```python
from build123d import *

# Parameters (mm, degrees)
F3_DEPTH = 34
F4_DEPTH = 18.001
F6_D     = 20
F7_R     = 7.5
F8_DEPTH = 5


with BuildPart() as f3:
    # F0 (on Front) → F3 (new body)
    with BuildSketch(Plane.XZ):
        Polygon((-55, 15), (-55, 0), (34, 0), (34, 18), (22, 18), (19, 15), align=None)
    extrude(amount=F3_DEPTH)

    # F1 (on Top) → F4 (intersect, through all)
    with BuildSketch(Plane.XY):
        Polygon((16, 0), (-55, 0), (-55, -10), (0, -34), (34, -34), (34, -24), (16, -24), align=None)
    extrude(amount=F4_DEPTH, mode=Mode.INTERSECT)

    # F5: F3 across plane


with BuildPart() as f3_1:
    add(f3.part)
    add(f3.part.mirror(Plane.XZ))

    # F6 (through all)
    with Locations(Plane(origin=(0, 0, 0), x_dir=(1, 0, 0), z_dir=(0, 0, -1))):
        with Locations((0, 0)):
            Hole(F6_D / 2)

    # F7 (on face) → F8 (cut)
    with BuildSketch(Plane.XY.offset(15)):
        with Locations((-45, 0)):
            Circle(F7_R)
    extrude(amount=-F8_DEPTH, mode=Mode.SUBTRACT)


solid = f3_1.part
```
The listing builds one solid part. Answer for the finished solid, in the listing's coordinates (mm). A direction names the side the tool comes from. Round coordinates to 2 decimals unless told otherwise and drop trailing zeros. Order: outer loops, then holes, each group sorted by start corner. A loop starts at its lowest first (then second) coordinate and runs counter-clockwise, first axis right, second up. Notation, with made-up numbers: (69, 12) -> (124, 12) arc R29 ccw to (124, 37) -> close; hole circle Ø6 at (30, 32.5). An arc over 180 degrees is marked (long way). Answer as CSV lines item,"result". Start each with the question number.
(1) The part is cut by section B-B (x = 23). Determine the outline of the cut face in (y, z), then the cut area to 3 significant figures.
(2) The part is cut by section A-A (y = 6). Determine the outline of the cut face in (x, z).
(3) A tool of negligible diameter and unlimited length cuts with its end or side. For faces 5 (the face through (34, -29, 9)), 6 (the face through (-17, 0, 15)), 7 (the face through (25, -24, 9)), from which of +Z, -Z, +X, -X, +Y, -Y can it reach the whole face along a straight path? Write none if from no direction.
(4) Flat-ended cylindrical pins translate along their axes: pin 1 Ø8 at (x, z) = (-36, 15) entering from +Y; pin 2 Ø12 at (x, y) = (0, 0) entering from +Z; pin 3 Ø20.5 at (x, y) = (-3, -13.5) entering from +Z; pin 4 Ø2 at (y, z) = (-26, 10.5) entering from -X (3 decimals). Find the tip coordinate at first contact, or state that the pin passes through.
(5) For a pull along X with two mould halves and no side action, classify faces 1 (the face through (-45, 0, 10)), 2 (the face through (28, 29, 18)), 3 (the face through (16, 0, 7)), 4 (the face through (-37.846, 2.253, 12.535)) as +X half, -X half, draft (parallel to the pull), parting line (faces both ways), or undercut.
(6) The part is cut by section D-D (z = 3). Determine the outline of the cut face in (x, y).
(7) The part is cut by section C-C (z = 13.75). Determine the outline of the cut face in (x, y).
(8) Find the intervals of material crossed by probe 1 along Y at (x, z) = (22.5, 13.5); probe 2 along Y at (x, z) = (0, 8); probe 3 along Z at (x, y) = (-9, 14), in increasing order. Write a range as from..to.
Evaluation:
1,outline,"(-34, 0) -> (-24, 0) -> (-24, 18) -> (-34, 18) -> close; (24, 0) -> (34, 0) -> (34, 18) -> (24, 18) -> close"
1,area,"360 mm²"
2,outline,"(-55, 0) -> (-8, 0) -> (-8, 15) -> (-40.5, 15) -> (-40.5, 10) -> (-49.5, 10) -> (-49.5, 15) -> (-55, 15) -> close; (8, 0) -> (16, 0) -> (16, 15) -> (8, 15) -> close"
3,face 5,"+Z, -Z, +X, +Y, -Y"
3,face 6,"+Z, -X, +Y, -Y"
3,face 7,"+Z, -Z, +X"
4,pin 1,"y = 20.04"
4,pin 2,"through"
4,pin 3,"z = 15"
4,pin 4,"x = -20.625"
5,face 1,"undercut"
5,face 2,"draft"
5,face 3,"+X half"
5,face 4,"undercut"
6,outline,"(-55, -10) -> (0, -34) -> (34, -34) -> (34, -24) -> (16, -24) -> (16, 24) -> (34, 24) -> (34, 34) -> (0, 34) -> (-55, 10) -> close; hole circle Ø20 at (0, 0)"
7,outline,"(-55, -10) -> (0, -34) -> (34, -34) -> (34, -24) -> (16, -24) -> (16, 24) -> (34, 24) -> (34, 34) -> (0, 34) -> (-55, 10) -> close; hole circle Ø15 at (-45, 0); hole circle Ø20 at (0, 0)"
8,probe 1,"-34..-24, 24..34"
8,probe 2,"-34..-10, 10..34"
8,probe 3,"0..15"
